Part model, mm, in its own coordinate system. Coordinates: 2 decimals unless noted, no trailing zeros. Order: outer loops, then holes, each group sorted by start corner. A loop starts at its lowest first (then second) coordinate and runs counter-clockwise, first axis right, second up.
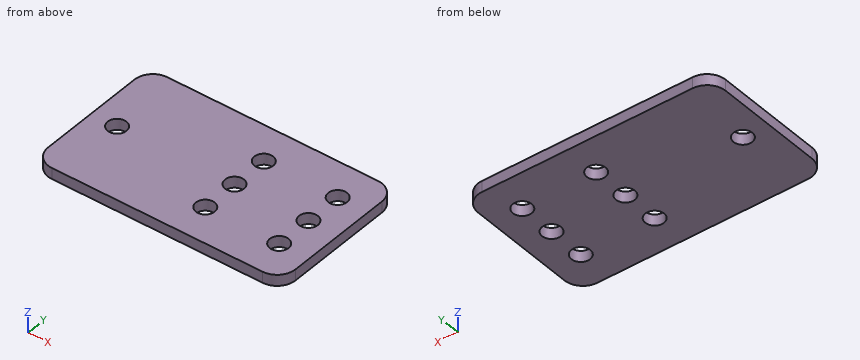
from build123d import *

# Parameters (mm, degrees)
SKETCH1_R           = 2.55
BOSS_EXTRUDE1_DEPTH = 1.5


with BuildPart() as part:
    # Sketch1 → Boss-Extrude1 (new body, symmetric)
    with BuildSketch(Plane.XY):
        with BuildLine():
            Line((-28.5, -19.75), (28.5, -19.75))
            ThreePointArc((28.5, -19.75), (32.035533906, -18.285533906), (33.5, -14.75))
            Line((33.5, -14.75), (33.5, 14.75))
            ThreePointArc((33.5, 14.75), (32.035533906, 18.285533906), (28.5, 19.75))
            Line((28.5, 19.75), (-28.5, 19.75))
            ThreePointArc((-28.5, 19.75), (-32.035533906, 18.285533906), (-33.5, 14.75))
            Line((-33.5, 14.75), (-33.5, -14.75))
            ThreePointArc((-33.5, -14.75), (-32.035533906, -18.285533906), (-28.5, -19.75))
        make_face()
        with Locations((5.29, 10)):
            Circle(SKETCH1_R, mode=Mode.SUBTRACT)
        with Locations((25.29, 10)):
            Circle(SKETCH1_R, mode=Mode.SUBTRACT)
        with Locations((5.29, 0)):
            Circle(SKETCH1_R, mode=Mode.SUBTRACT)
        with Locations((25.29, 0)):
            Circle(SKETCH1_R, mode=Mode.SUBTRACT)
        with Locations((5.29, -10)):
            Circle(SKETCH1_R, mode=Mode.SUBTRACT)
        with Locations((25.29, -10)):
            Circle(SKETCH1_R, mode=Mode.SUBTRACT)
        with Locations((-26.5, 0)):
            Circle(SKETCH1_R, mode=Mode.SUBTRACT)
    extrude(amount=BOSS_EXTRUDE1_DEPTH, both=True)


solid = part.part
Q1. Pin check, flat tip, straight feed: pin 1 Ø6 at (x, y) = (-26.5, 0) entering from +Z. Stop position of the tip, or through.
Results list:
pin 1: stops at z = 1.5
Q2. Cut at C-C on x = 5.29. Write the cut outline in (y, z).
Results list:
outline: (-19.75, -1.5) - (-12.55, -1.5) - (-12.55, 1.5) - (-19.75, 1.5) - close; (-7.45, -1.5) - (-2.55, -1.5) - (-2.55, 1.5) - (-7.45, 1.5) - close; (2.55, -1.5) - (7.45, -1.5) - (7.45, 1.5) - (2.55, 1.5) - close; (12.55, -1.5) - (19.75, -1.5) - (19.75, 1.5) - (12.55, 1.5) - close
Q3. Wall check: line 1 along Y through (x, z) = (25.5, 0.8); line 2 along Y through (x, z) = (26, 0.8); line 3 along X through (y, z) = (9.5, 0.4). Give the ranges that are in metal, low to high.
Results list:
line 1: y = -19.75 to -12.54, -7.46 to -2.54, 2.54 to 7.46, 12.54 to 19.75
line 2: y = -19.75 to -12.45, -7.55 to -2.45, 2.45 to 7.55, 12.45 to 19.75
line 3: x = -33.5 to 2.79, 7.79 to 22.79, 27.79 to 33.5
Q4. Cut at B-B on z = -0.05. Write the cut outline in (x, y).
Results list:
outline: (-33.5, -14.75) arc R5 ccw to (-28.5, -19.75) - (28.5, -19.75) arc R5 ccw to (33.5, -14.75) - (33.5, 14.75) arc R5 ccw to (28.5, 19.75) - (-28.5, 19.75) arc R5 ccw to (-33.5, 14.75) - close; hole circle Ø5.1 at (-26.5, 0); hole circle Ø5.1 at (5.29, -10); hole circle Ø5.1 at (5.29, 0); hole circle Ø5.1 at (5.29, 10); hole circle Ø5.1 at (25.29, -10); hole circle Ø5.1 at (25.29, 0); hole circle Ø5.1 at (25.29, 10)
Q5. Cut at A-A on y = 0. Write the cut outline in (x, z).
Results list:
outline: (-33.5, -1.5) - (-29.05, -1.5) - (-29.05, 1.5) - (-33.5, 1.5) - close; (-23.95, -1.5) - (2.74, -1.5) - (2.74, 1.5) - (-23.95, 1.5) - close; (7.84, -1.5) - (22.74, -1.5) - (22.74, 1.5) - (7.84, 1.5) - close; (27.84, -1.5) - (33.5, -1.5) - (33.5, 1.5) - (27.84, 1.5) - close
Q6. Cut at D-D on y = -10. Write the cut outline in (x, z).
Results list:
outline: (-33.5, -1.5) - (2.74, -1.5) - (2.74, 1.5) - (-33.5, 1.5) - close; (7.84, -1.5) - (22.74, -1.5) - (22.74, 1.5) - (7.84, 1.5) - close; (27.84, -1.5) - (33.5, -1.5) - (33.5, 1.5) - (27.84, 1.5) - close
